Can you work these out from the drawing? Everything is in mm from the part's minimum corner. Give positions to 0.01 mm unless a question says otherwise; leave off trailing zeros. Write each loop counter-clockwise with the first axis right and the second up, starting at its lowest first coordinate (ties: lowest second). Pieces come first, ordered by that corner, then holes. Notation, with made-up numbers: (6.25, 43.25) - (30.25, 43.25) arc R24 cw to (30.25, 57.25) - close; hole circle Ø2 at (12, 61). An arc over 180 degrees is marked (long way). Use a Markdown table: item, result.
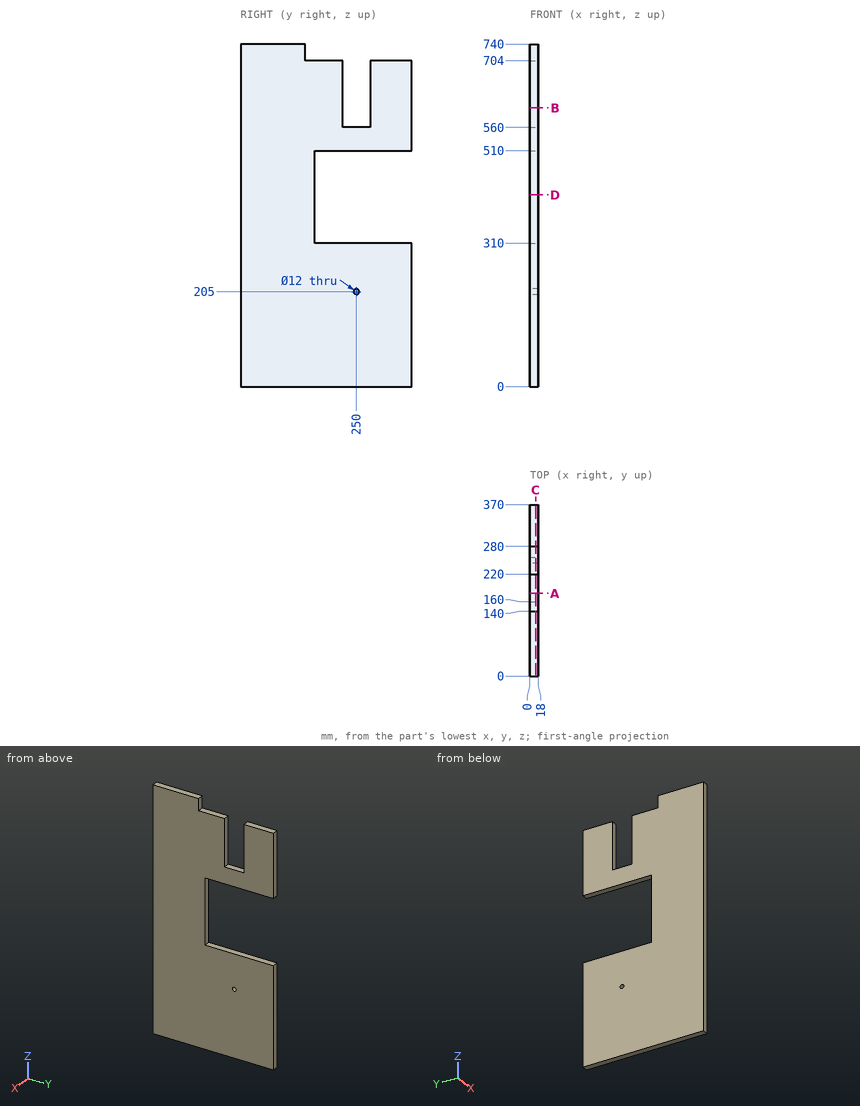
Item 1: If we section it at B-B, the plane z = 602: Write out the boundary of the cut face in (x, y).
Values:
| item | result |
|---|---|
| outline | (0, 0) - (18, 0) - (18, 220) - (0, 220) - close; (0, 280) - (18, 280) - (18, 370) - (0, 370) - close |
Item 2: If we section it at C-C, the plane x = 12: Write out the boundary of the cut face in (y, z), plus the area to 3 significant figures.
Values:
| item | result |
|---|---|
| outline | (0, 0) - (370, 0) - (370, 310) - (160, 310) - (160, 510) - (370, 510) - (370, 704) - (280, 704) - (280, 560) - (220, 560) - (220, 704) - (140, 704) - (140, 740) - (0, 740) - close; hole circle Ø12 at (250, 205) |
| area | 215,000 mm2 |
Item 3: If we section it at D-D, the plane z = 414: Write out the boundary of the cut face in (x, y), plus the area to 3 significant figures.
Values:
| item | result |
|---|---|
| outline | (0, 0) - (18, 0) - (18, 160) - (0, 160) - close |
| area | 2,880 mm2 |
Item 4: If we section it at A-A, the plane y = 178.5: Write out the boundary of the cut face in (x, z).
Values:
| item | result |
|---|---|
| outline | (0, 0) - (18, 0) - (18, 310) - (0, 310) - close; (0, 510) - (18, 510) - (18, 704) - (0, 704) - close |
Item 5: I need wall thicknesses on line 1 along Z through (x, y) = (12, 250); line 2 along Z through (x, y) = (1.25, 348.5); line 3 along Y through (x, z) = (9.25, 581). Which ranges of each line are inside material? Lowest first, please. Write a range as [from, to].
Values:
| item | result |
|---|---|
| line 1 | z = [0, 199], [211, 310], [510, 560] |
| line 2 | z = [0, 310], [510, 704] |
| line 3 | y = [0, 220], [280, 370] |
Item 6: Will these pins go through, and if not, where does the flat tip stop? pin 1 Ø5.5 at (x, y) = (9.5, 261) entering from +Z; pin 2 Ø9 at (x, y) = (5, 286.5) entering from +Z.
Values:
| item | result |
|---|---|
| pin 1 | stops at z = 560 |
| pin 2 | stops at z = 704 |
